Build history of the part. All positions in model axes, mm. Face numbers are marked on the shaded views. A direction names the side the tool comes from. Round coordinates to 2 decimals unless told otherwise and drop trailing zeros. Order: outer loops, then holes, each group sorted by start corner. A loop starts at its lowest first (then second) coordinate and runs counter-clockwise, first axis right, second up. Notation, with made-up numbers: (12, 70.25) -> (19, 70.25) arc R30 cw to (19, 100.25) -> close; hole circle Ø11 at (50.25, -1.5). An arc over 180 degrees is marked (long way). Answer as a JSON object with one key per item and string values.
from build123d import *

# Parameters (mm, degrees)
F1_DEPTH = 10
F2_R     = 1
F3_DEPTH = 52.9
F4_R     = 1
F5_DEPTH = 41.9


with BuildPart() as f1:
    # F0 (on Front) → F1 (new body)
    with BuildSketch(Plane.XZ):
        Polygon((-60, -10), (-60, -25), (50, -25), (50, -10), (60, -10), (60, 10), (50, 10), (50, 25), (-60, 25), (-60, 10), (-50, 10), (-50, -10), align=None)
    extrude(amount=F1_DEPTH)

    # F2 (on face) → F3 (cut)
    with BuildSketch(Plane(origin=(0, 0, -25), x_dir=(1, 0, 0), z_dir=(0, 0, -1))):
        with Locations((-55, 5)):
            Circle(F2_R)
    extrude(amount=-F3_DEPTH, mode=Mode.SUBTRACT)

    # F4 (on face) → F5 (cut)
    with BuildSketch(Plane(origin=(0, 0, -10), x_dir=(1, 0, 0), z_dir=(0, 0, -1))):
        with Locations((55, 5)):
            Circle(F4_R)
    extrude(amount=-F5_DEPTH, mode=Mode.SUBTRACT)


solid = f1.part
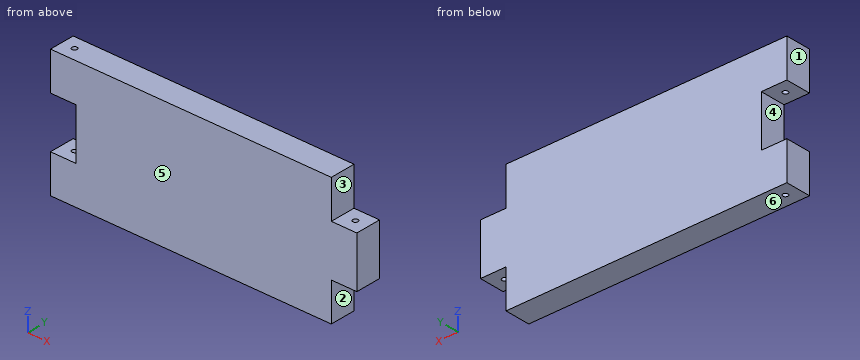
1) Probe L1, parallel to Y at x = 55, z = -5.25; L2, parallel to X at y = -5, z = 1.75; L3, parallel to X at y = -5, z = -15. List the from-to ranges inside material, lowest first. Write a range as from..to.
Checked values:
{"L1": "y = -10..-6, -4..0", "L2": "x = -50..54, 56..60", "L3": "x = -60..-56, -54..50"}
2) Cut at A-A, the plane z = -1. Give the cut face in (x, y).
Checked values:
{"outline": "(-50, -10) -> (60, -10) -> (60, 0) -> (-50, 0) -> close; hole circle Ø2 at (55, -5)"}
3) Pull direction Z, two halves, no side cores. Call the marked faces 4, 5 and 6: pulls with the +Z half, pulls with the -Z half, needs draft (parallel to the pull), parting line crosses it, or undercut.
Checked values:
{"face 4": "undercut", "face 5": "needs draft", "face 6": "pulls with the -Z half"}
4) Cut at B-B, the plane y = -8.75. Give the cut face in (x, z).
Checked values:
{"outline": "(-60, -25) -> (50, -25) -> (50, -10) -> (60, -10) -> (60, 10) -> (50, 10) -> (50, 25) -> (-60, 25) -> (-60, 10) -> (-50, 10) -> (-50, -10) -> (-60, -10) -> close"}
5) Flat gauge pins, fed straight in: pin 1 Ø2.5 at (x, y) = (55, -5) entering from -Z; pin 2 Ø1.6 at (x, y) = (-55, -5) entering from -Z; pin 3 Ø3 at (y, z) = (-7.5, -20) entering from +X; pin 4 Ø3 at (x, y) = (53.5, -7) entering from +Z. Where does each tip first touch, or does it go through?
Checked values:
{"pin 1": "stops at z = -10", "pin 2": "passes through", "pin 3": "stops at x = 50", "pin 4": "stops at z = 10"}
6) Which spindle directions (+Z, -Z, +X, -X, +Y, -Y) get a long thin tool onto all of the face, cutting with end or side? Do the marked faces 1, 2 and 3. Say none if no direction does.
Checked values:
{"face 1": "+Z, -Z, -X, +Y, -Y", "face 2": "-Z, +X, +Y, -Y", "face 3": "+Z, +X, +Y, -Y"}
